Autodesk Inventor part; units mm, degrees
ref_plane "YZ Plane" through (0, 0, 0) normal (1, 0, 0) x (0, 1, 0)
ref_plane "XZ Plane" through (0, 0, 0) normal (0, 1, 0) x (-1, 0, 0)
ref_plane "XY Plane" through (0, 0, 0) normal (0, 0, 1) x (1, 0, 0)
sketch "草圖1" plane through (0, 0, 0) normal (0, 1, 0) x (-1, 0, 0)
  line L0 (8.5, 8.5) -> (-8.5, 8.5)
  line L1 (-8.5, 8.5) -> (-8.5, -8.5)
  line L2 (-8.5, -8.5) -> (8.5, -8.5)
  line L3 (8.5, -8.5) -> (8.5, 8.5)
  line L4 (8.5, 8.5) -> (-8.5, -8.5) construction
  line L5 (-8.5, 8.5) -> (8.5, -8.5) construction
  point P0 (0, 0)
  dimension "d0" = 17
  dimension "d1" = 17
extrude "擠出1" add sketch "草圖1" along normal blind 2
sketch "草圖3" plane through (0, 0, 0) normal (0, -1, 0) x (1, 0, 0)
  line L0 (-4.4, 2.5) -> (-2.5, 2.5)
  line L1 (-2.5, 2.5) -> (-2.5, -2.5)
  line L2 (-2.5, -2.5) -> (-4.4, -2.5)
  line L3 (-4.4, -2.5) -> (-4.4, 2.5)
  line L4 (-4.4, 2.5) -> (-2.5, -2.5) construction
  line L5 (-2.5, 2.5) -> (-4.4, -2.5) construction
  line L6 (2.5, 2.5) -> (4.4, 2.5)
  line L7 (4.4, 2.5) -> (4.4, -2.5)
  line L8 (4.4, -2.5) -> (2.5, -2.5)
  line L9 (2.5, -2.5) -> (2.5, 2.5)
  line L10 (2.5, 2.5) -> (4.4, -2.5) construction
  line L11 (4.4, 2.5) -> (2.5, -2.5) construction
  point P0 (0, 0)
  point P1 (-3.45, 0)
  point P2 (3.45, 0)
  dimension "d4" = 1.9
  dimension "d5" = 1.9
  dimension "d6" = 5
  dimension "d7" = 5
  dimension "d8" = 0
  dimension "d9" = 5
  dimension "d10" = 2.5
extrude "擠出2" add sketch "草圖3" along normal blind 1
sketch "草圖4" plane through (0, 0, 0) normal (0, -1, 0) x (1, 0, 0)
  line L0 (-8.5, -8.5) -> (-8.5, 8.5)
  line L1 (8.5, 8.5) -> (8.5, -8.5)
  line L2 (-8.5, 8.5) -> (8.5, 8.5)
  line L3 (8.5, 8.5) -> (8.5, 7.5)
  line L4 (8.5, 7.5) -> (-8.5, 7.5)
  line L5 (-8.5, 7.5) -> (-8.5, 8.5)
  line L6 (-8.5, -7.5) -> (8.5, -7.5)
  line L7 (8.5, -7.5) -> (8.5, -8.5)
  line L8 (8.5, -8.5) -> (-8.5, -8.5)
  line L9 (-8.5, -8.5) -> (-8.5, -7.5)
  point P0 (0, 0)
  point P1 (-8.5, -7.5)
  point P2 (-8.5, 7.5)
  dimension "d13" = 1
  dimension "d14" = 1
extrude "擠出3" add sketch "草圖4" along normal blind 5 contours L0 L6 L1 L8 | L0 L2 L1 L4
sketch "草圖5" plane through (8.5, 0, 7.5) normal (0, 0, -1) x (-1, 0, 0)
  line L0 (10.5, -12) -> (6.5, -12)
  line L1 (6.5, -12) -> (6.5, 2)
  line L2 (6.5, 2) -> (10.5, 2)
  line L3 (10.5, 2) -> (10.5, -12)
  line L4 (0, -5) -> (17, -5)
  line L5 (10.5, -12) -> (6.5, 2) construction
  line L6 (6.5, -12) -> (10.5, 2) construction
  point P0 (8.5, 0)
  point P1 (8.5, -5)
  point P2 (6.5, -5)
  point P3 (10.5, -5)
  dimension "d17" = 14
  dimension "d18" = 4
extrude "擠出4" add sketch "草圖5" along normal blind 1.5 contours L4 L1 L2 L3
sketch "草圖6" plane through (-8.5, 0, -7.5) normal (0, 0, 1) x (1, 0, 0)
  line L0 (6.5, 2) -> (10.5, 2)
  line L1 (10.5, 2) -> (10.5, -12)
  line L2 (10.5, -12) -> (6.5, -12)
  line L3 (6.5, -12) -> (6.5, 2)
  line L4 (10.5, -5) -> (6.5, -5)
  line L5 (6.5, 2) -> (10.5, -12) construction
  line L6 (10.5, 2) -> (6.5, -12) construction
  point P0 (8.5, 0)
  point P1 (8.5, -5)
  point P2 (10.5, -7)
  point P3 (6.5, -7)
  dimension "d21" = 14
  dimension "d22" = 4
extrude "擠出5" add sketch "草圖6" along normal blind 1.5 contours L0 L1 L4 L3
sketch "草圖7" plane through (0, 2, 0) normal (0, 1, 0) x (1, 0, 0)
  line L0 (-2.5, 6) -> (2.5, 6)
  line L1 (2.5, 6) -> (2.5, -6)
  line L2 (2.5, -6) -> (-2.5, -6)
  line L3 (-2.5, -6) -> (-2.5, 6)
  line L4 (-2.5, 6) -> (2.5, -6) construction
  line L5 (2.5, 6) -> (-2.5, -6) construction
  point P0 (0, 0)
  dimension "d25" = 12
  dimension "d26" = 5
extrude "擠出6" add sketch "草圖7" along normal blind 25
sketch "草圖8" plane through (-2.5, 2, -6) normal (-1, 0, 0) x (0, 0, 1)
  circle A0 centre (6, 20) radius 2.6
  circle A1 centre (6, 10) radius 2.6
  line L0 (-2.5, 0) -> (14.5, 0)
  point P0 (6, -2)
  point P1 (6, 0)
  dimension "d29" = 5.2
  dimension "d30" = 5.2
  dimension "d31" = 10
  dimension "d32" = 10
extrude "擠出7" cut sketch "草圖8" against normal blind 25
properties part number "差分線圈上蓋"
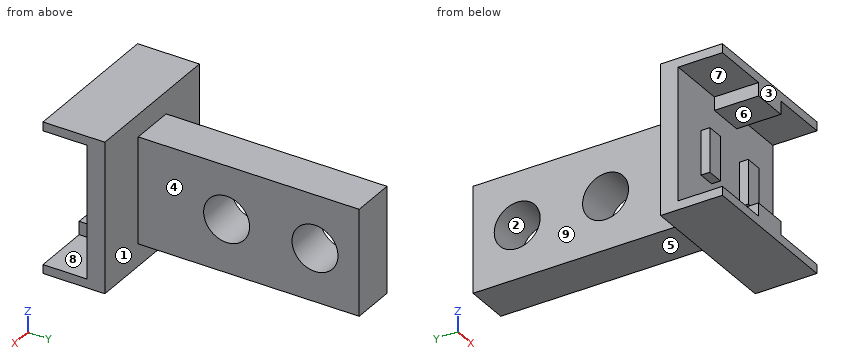
Work out the finished part from the listing and answer in its coordinate system (mm). Face numbers are marked on the shaded views. A direction names the side the tool comes from. Round coordinates to 2 decimals unless told otherwise and drop trailing zeros. Loops run counter-clockwise (first coordinate to the right, second up) from the corner with the lowest first, then second, coordinate; pieces in that order, holes last. Notation, with made-up numbers: (17.25, 83) - (30.25, 83) arc R28 cw to (30.25, 119) - close; hole circle Ø1 at (76.25, 33). An arc over 180 degrees is marked (long way). One line per item, written item: value.
Q1. The mould has two halves that part along Y. Classify the marked faces 1, 2, 3 and 4: +Y half, -Y half, draft (parallel to the pull), parting line (faces both ways), or undercut.
Check values:
face 1: +Y half
face 2: undercut
face 3: -Y half
face 4: draft
Q2. Find section C-C on x = -5.75. Give the vertices of the cut face in (y, z).
Check values:
outline: (-5, -8.5) - (2, -8.5) - (2, 8.5) - (-5, 8.5) - (-5, 7.5) - (0, 7.5) - (0, -7.5) - (-5, -7.5) - close
Q3. For the marked faces 5, 6, 7, 8 and 9, determine the directions among +Z, -Z, +X, -X, +Y, -Y from which every point of the face is accessible in a straight line to the end or side of a thin tool.
Check values:
face 5: -Z, +X, -X, +Y
face 6: +X, -X, -Y
face 7: -X, -Y
face 8: +X, -Y
face 9: +Z, -Z, -X, +Y
Q4. Straight lines are drawn through the part: probe 1 along Y at (x, z) = (1.4, 0); probe 2 along Y at (x, z) = (0.5, -2); probe 3 along X at (y, z) = (25.5, 2.25). For each, find the intervals that lie inside material, in ascending order.
Check values:
probe 1: 0 to 9.4, 14.6 to 19.4, 24.6 to 27
probe 2: 0 to 10.34, 13.66 to 20.34, 23.66 to 27
probe 3: -2.5 to 2.5
Q5. Find section D-D on x = 0.5. Give the vertices of the cut face in (y, z), and give its area (3 significant figures).
Check values:
outline: (-5, -8.5) - (2, -8.5) - (2, -6) - (27, -6) - (27, 6) - (2, 6) - (2, 8.5) - (-5, 8.5) - (-5, 6) - (0, 6) - (0, -6) - (-5, -6) - close; hole circle Ø5.2 at (12, 0); hole circle Ø5.2 at (22, 0)
area: 317 mm2
Q6. Find section B-B on y = -2. Give the vertices of the cut face in (x, z), and give its area (3 significant figures).
Check values:
outline: (-8.5, -8.5) - (8.5, -8.5) - (8.5, -7.5) - (2, -7.5) - (2, -6) - (-2, -6) - (-2, -7.5) - (-8.5, -7.5) - close; (-8.5, 7.5) - (-2, 7.5) - (-2, 6) - (2, 6) - (2, 7.5) - (8.5, 7.5) - (8.5, 8.5) - (-8.5, 8.5) - close
area: 46.0 mm2
Q7. Find section A-A on z = 0. Give the vertices of the cut face in (x, y).
Check values:
outline: (-8.5, 0) - (-4.4, 0) - (-4.4, -1) - (-2.5, -1) - (-2.5, 0) - (2.5, 0) - (2.5, -1) - (4.4, -1) - (4.4, 0) - (8.5, 0) - (8.5, 2) - (2.5, 2) - (2.5, 9.4) - (-2.5, 9.4) - (-2.5, 2) - (-8.5, 2) - close; (-2.5, 14.6) - (2.5, 14.6) - (2.5, 19.4) - (-2.5, 19.4) - close; (-2.5, 24.6) - (2.5, 24.6) - (2.5, 27) - (-2.5, 27) - close
Q8. Each of these flat-tipped pins is pushed along its axis until it touches: pin 1 Ø4.5 at (y, z) = (22, 0) entering from -X; pin 2 Ø0.5 at (y, z) = (-0.5, -0.5) entering from -X; pin 3 Ø4 at (y, z) = (8.5, 5.5) entering from -X; pin 4 Ø1 at (x, y) = (0.5, 22) entering from +Z. Where does it stop, or does it pass through?
Check values:
pin 1: through
pin 2: x = -4.4
pin 3: x = -2.5
pin 4: z = 6
